Part model, mm, in its own coordinate system. Round coordinates to 2 decimals unless told otherwise and drop trailing zeros. Order: outer loops, then holes, each group sorted by start corner. A loop starts at its lowest first (then second) coordinate and runs counter-clockwise, first axis right, second up. Notation, with made-up numbers: (84.25, 46) -> (132.25, 46) arc R10 cw to (132.25, 51) -> close; hole circle Ø8 at (-20.5, 35.25). An arc over 180 degrees is marked (long way). Answer as a JSON object with one key per item and string values. Group by question number.
```python
from build123d import *

# Parameters (mm, degrees)
F0_R     = 6.6
F0_R_2   = 6.55
F1_DEPTH = 5


with BuildPart() as f1:
    # F0 (on Top) → F1 (new body)
    with BuildSketch(Plane.XY):
        with BuildLine():
            Line((16.15, 10.01215), (0, 10.01215))
            ThreePointArc((0, 10.01215), (-6.6731, 7.538008), (-10.120357, 1.311607))
            ThreePointArc((-10.120357, 1.311607), (-8.866222, -0.208711), (-10.125611, -1.724678))
            ThreePointArc((-10.125611, -1.724678), (-6.686523, -7.974556), (0, -10.460258))
            Line((0, -10.460258), (16.15, -10.460258))
            ThreePointArc((16.15, -10.460258), (26.386204, -0.224054), (16.15, 10.01215))
        make_face()
        Circle(F0_R, mode=Mode.SUBTRACT)
        with Locations((16.15, 0)):
            Circle(F0_R_2, mode=Mode.SUBTRACT)
    extrude(amount=F1_DEPTH)


solid = f1.part
```
Q1. Band-saw the part on C-C (x = -5). List the corners of the cut face in (y, z), plus the area to 3 significant figures.
Q2. Wall check: line 1 (Y direction, x = 0, z = 1.5); line 2 (X direction, y = 4, z = 3.05); line 3 (Y direction, x = 16.15, z = 3.7). Give the ranges that are in metal, low to high. Write a range as [from, to].
Q3. Drop flat-ended pins along their axis: pin 1 Ø1 at (y, z) = (5.5, 4) entering from +X; pin 2 Ø1.5 at (y, z) = (5, 1) entering from -X. Give the stop position or say it passes through.
Q4. Band-saw the part on B-B (y = 0). List the corners of the cut face in (x, z), plus the area to 3 significant figures.
Q5. Two-plate mould, pull along Y, no slides. Class faces 1 (the cylindrical face through (26.384, -0.449, 2.465)), 2 (the cylindrical face through (19.671, 5.523, 2.465)), 3 (the flat face through (8, -10.46, 2)), 4 (the cylindrical face through (-4.864, 4.461, 2.465)): +Y half, -Y half, draft (parallel to the pull), parting line (faces both ways), or undercut.
Q6. Band-saw the part on D-D (y = -3). List the corners of the cut face in (x, z), plus the area to 3 significant figures.
Completed:
{
 "1": {"outline": "(-9.16, 0) -> (-4.31, 0) -> (-4.31, 5) -> (-9.16, 5) -> close; (4.31, 0) -> (8.71, 0) -> (8.71, 5) -> (4.31, 5) -> close", "area": "46.2 mm2"},
 "2": {"line 1": "[-10.46, -6.6], [6.6, 10.01]", "line 2": "[-9.32, -5.25], [5.25, 10.96], [21.34, 25.47]", "line 3": "[-10.46, -6.55], [6.55, 10.01]"},
 "3": {"pin 1": "x = 24.95", "pin 2": "x = -9.21"},
 "4": {"outline": "(-8.88, 0) -> (-6.6, 0) -> (-6.6, 5) -> (-8.88, 5) -> close; (6.6, 0) -> (9.6, 0) -> (9.6, 5) -> (6.6, 5) -> close; (22.7, 0) -> (26.38, 0) -> (26.38, 5) -> (22.7, 5) -> close", "area": "44.8 mm2"},
 "5": {"face 1": "parting line", "face 2": "undercut", "face 3": "-Y half", "face 4": "undercut"},
 "6": {"outline": "(-9.85, 0) -> (-5.88, 0) -> (-5.88, 5) -> (-9.85, 5) -> close; (5.88, 0) -> (10.33, 0) -> (10.33, 5) -> (5.88, 5) -> close; (21.97, 0) -> (26, 0) -> (26, 5) -> (21.97, 5) -> close", "area": "62.3 mm2"}
}
